Check sheet for the modelled part. Datum: model origin and axes. Units: mm. A direction names the side the tool comes from. Round coordinates to 2 decimals unless told otherwise and drop trailing zeros. Loops run counter-clockwise (first coordinate to the right, second up) from the corner with the lowest first, then second, coordinate; pieces in that order, holes last. Notation, with made-up numbers: (67, -28.5) - (81, -28.5) arc R19 cw to (81, -23.5) - close; hole circle Ø3 at (-17, 79). An arc over 180 degrees is marked (long way). Put each result on its own line as item: value.
```python
from build123d import *

# Parameters (mm, degrees)
BASE_FLANGE1_DEPTH      = 304.8
CUT_EXTRUDE1_DEPTH      = 408.166225608
CUT_EXTRUDE1_DEPTH_BACK = 408.166225608
SKETCH6_W               = 152.4
SKETCH6_H               = 12.7
EDGE_FLANGE1_DEPTH      = 521.87348
EDGE_FLANGE1_BEND_DEPTH = 521.87348
F_1_4_CLEARANCE_HOLE1_D = 6.7564
FILLET1_R               = 2.54
CUT_EXTRUDE2_DEPTH      = 412.498279143
CUT_EXTRUDE3_DEPTH      = 412.769633365
FILLET2_R               = 1.27


# Sheet-metal steps are written as plain solids
with BuildPart() as part:
    # Sketch1 → Base-Flange1 (new body)
    with BuildSketch(Plane(origin=(0, 0, 0), x_dir=(0, 0, -1), z_dir=(1, 0, 0))):
        with BuildLine():
            Line((-266.7, 44.45), (-266.7, 5.76326))
            ThreePointArc((-266.7, 5.76326), (-265.011980228, 1.688019772), (-260.93674, 0))
            Line((-260.93674, 0), (260.93674, 0))
            ThreePointArc((260.93674, 0), (265.011980228, 1.688019772), (266.7, 5.76326))
            Line((266.7, 5.76326), (266.7, 44.45))
            Line((266.7, 44.45), (264.11174, 44.45))
            Line((264.11174, 44.45), (264.11174, 5.76326))
            ThreePointArc((264.11174, 5.76326), (263.18180403, 3.51819597), (260.93674, 2.58826))
            Line((260.93674, 2.58826), (-260.93674, 2.58826))
            ThreePointArc((-260.93674, 2.58826), (-263.18180403, 3.51819597), (-264.11174, 5.76326))
            Line((-264.11174, 5.76326), (-264.11174, 44.45))
            Line((-264.11174, 44.45), (-266.7, 44.45))
        make_face()
    extrude(amount=BASE_FLANGE1_DEPTH)

    # Sketch6 → Cut-Extrude1 (cut, two sides: drawn at the far end of the back side and taken through both)
    with BuildSketch(Plane(origin=(0, 2.58826, 0), x_dir=(1, 0, 0), z_dir=(0, 1, 0)).offset(-CUT_EXTRUDE1_DEPTH_BACK)):
        with Locations((152.4, 260.35)):
            Rectangle(SKETCH6_W, SKETCH6_H)
        with Locations((152.4, -260.35)):
            Rectangle(SKETCH6_W, SKETCH6_H)
    extrude(amount=CUT_EXTRUDE1_DEPTH + CUT_EXTRUDE1_DEPTH_BACK, mode=Mode.SUBTRACT)

    # Edge-Flange1 section (across the edge) → Edge-Flange1 (add)
    with BuildSketch(Plane(origin=(-3.175, 2.58826, -260.93674), x_dir=(1, 0, 0), z_dir=(0, 0, 1))):
        with BuildLine():
            Line((-2.58826, 3.175), (-2.58826, 29.16174))
            Line((-2.58826, 29.16174), (0, 29.16174))
            Line((0, 29.16174), (0, 3.175))
            ThreePointArc((0, 3.175), (0.92993597, 0.92993597), (3.175, 0))
            Line((3.175, 0), (3.175, -2.58826))
            ThreePointArc((3.175, -2.58826), (-0.900240228, -0.900240228), (-2.58826, 3.175))
        make_face()
    extrude(amount=EDGE_FLANGE1_DEPTH)

    # Edge-Flange1 section 2 (across the edge) → Edge-Flange1 bend (add)
    with BuildSketch(Plane(origin=(307.975, 2.58826, 260.93674), x_dir=(-1, 0, 0), z_dir=(0, 0, -1))):
        with BuildLine():
            Line((-2.58826, 3.175), (-2.58826, 29.16174))
            Line((-2.58826, 29.16174), (0, 29.16174))
            Line((0, 29.16174), (0, 3.175))
            ThreePointArc((0, 3.175), (0.92993597, 0.92993597), (3.175, 0))
            Line((3.175, 0), (3.175, -2.58826))
            ThreePointArc((3.175, -2.58826), (-0.900240228, -0.900240228), (-2.58826, 3.175))
        make_face()
    extrude(amount=EDGE_FLANGE1_BEND_DEPTH)

    # 1/4 Clearance Hole1 (through all)
    with Locations(Plane.XY.offset(266.7)):
        with Locations((38.1, 31.75), (266.7, 31.75)):
            Hole(F_1_4_CLEARANCE_HOLE1_D / 2)

    # Fillet1
    fillet1_edges = [part.edges().sort_by_distance(p)[0] for p in [
        (0, 44.45, 265.40587),
        (-4.46913, 31.75, -260.93674),
        (-4.46913, 31.75, 260.93674),
        (0, 44.45, -265.40587),
        (309.26913, 31.75, 260.93674),
        (309.26913, 31.75, -260.93674),
        (304.8, 44.45, 265.40587),
        (76.2, 1.29413, -254),
        (228.6, 1.29413, -254),
        (228.6, 44.45, -265.40587),
        (76.2, 44.45, -265.40587),
        (304.8, 44.45, -265.40587),
        (228.6, 1.29413, 254),
        (76.2, 1.29413, 254),
        (76.2, 44.45, 265.40587),
        (228.6, 44.45, 265.40587),
    ]]
    fillet(fillet1_edges, radius=FILLET1_R)

    # Sketch15 → Cut-Extrude2 (cut, through all)
    with BuildSketch(Plane(origin=(0, 2.58826, 0), x_dir=(1, 0, 0), z_dir=(0, 1, 0))):
        with BuildLine():
            Line((149.86, 22.86), (149.86, 2.54))
            Line((149.86, 2.54), (129.54, 2.54))
            ThreePointArc((129.54, 2.54), (127, 0), (129.54, -2.54))
            Line((129.54, -2.54), (149.86, -2.54))
            Line((149.86, -2.54), (149.86, -22.86))
            ThreePointArc((149.86, -22.86), (152.4, -25.4), (154.94, -22.86))
            Line((154.94, -22.86), (154.94, -2.54))
            Line((154.94, -2.54), (175.26, -2.54))
            ThreePointArc((175.26, -2.54), (177.8, 0), (175.26, 2.54))
            Line((175.26, 2.54), (154.94, 2.54))
            Line((154.94, 2.54), (154.94, 22.86))
            ThreePointArc((154.94, 22.86), (152.4, 25.4), (149.86, 22.86))
        make_face()
    extrude(amount=-CUT_EXTRUDE2_DEPTH, mode=Mode.SUBTRACT)

    # Sketch16 → Cut-Extrude3 (cut, through all)
    with BuildSketch(Plane.XZ):
        with BuildLine():
            Line((149.86, -254), (149.86, -231.14))
            ThreePointArc((149.86, -231.14), (152.4, -228.6), (154.94, -231.14))
            Line((154.94, -231.14), (154.94, -254))
            Line((154.94, -254), (149.86, -254))
        make_face()
        with BuildLine():
            Line((154.94, 254), (149.86, 254))
            Line((149.86, 254), (149.86, 231.14))
            ThreePointArc((149.86, 231.14), (152.4, 228.6), (154.94, 231.14))
            Line((154.94, 231.14), (154.94, 254))
        make_face()
    extrude(amount=-CUT_EXTRUDE3_DEPTH, mode=Mode.SUBTRACT)

    # Fillet2
    fillet2_edges = [part.edges().sort_by_distance(p)[0] for p in [
        (149.86, 1.29413, -2.54),
        (154.94, 1.29413, -2.54),
        (154.94, 1.29413, 2.54),
        (149.86, 1.29413, 2.54),
        (154.94, 1.29413, 254),
        (149.86, 1.29413, 254),
        (154.94, 1.29413, -254),
        (149.86, 1.29413, -254),
    ]]
    fillet(fillet2_edges, radius=FILLET2_R)


solid = part.part
```
Item 1: Section check C-C on z = 221.5. Enter the section's corners in (x, y) (3 decimals), then the cut area to 3 significant figures.
Filled sheet:
outline: (-5.763, 5.763) arc R5.763 ccw to (0, 0) - (304.8, 0) arc R5.763 ccw to (310.563, 5.763) - (310.563, 31.75) - (307.975, 31.75) - (307.975, 5.763) arc R3.175 cw to (304.8, 2.588) - (0, 2.588) arc R3.175 cw to (-3.175, 5.763) - (-3.175, 31.75) - (-5.763, 31.75) - close
area: 960 mm²
Item 2: Thickness scan on line 1 (X direction, y = 27, z = -184.5) (3 decimals); line 2 (X direction, y = 31, z = 265); line 3 (Z direction, x = 68, y = 15). Record the ranges inside material, lowest first. Write a range as from..to.
Filled sheet:
line 1: -5.763..-3.175, 307.975..310.563
line 2: 0..34.81, 41.39..76.2, 228.6..263.41, 269.99..304.8
line 3: -266.7..-264.11, 264.11..266.7
Item 3: Tool access check on faces 5 (the flat face through (228.6, 18, 265)), 6 (the flat face through (-5.763, 19, -4)), 7 (the flat face through (307.975, 19, 4)), 8 (the flat face through (38, 25, 264.112)), 9 (the flat face through (76.2, 18, -265)). Record the directions out of +Z, -Z, +X, -X, +Y, -Y that give a thin tool (end or side, any length) a straight path to the whole face; none if there is none.
Filled sheet:
face 5: +Z, +Y, -Y
face 6: +Z, -Z, -X, +Y, -Y
face 7: +Z, -Z, +Y
face 8: +X, -X, +Y
face 9: -Z, +Y, -Y
Item 4: Section check A-A on y = 16.5. Enter the section's corners in (x, z) (3 decimals).
Filled sheet:
outline: (-5.763, -260.937) - (-3.175, -260.937) - (-3.175, 260.937) - (-5.763, 260.937) - close; (0, -266.7) - (76.2, -266.7) - (76.2, -264.112) - (0, -264.112) - close; (0, 264.112) - (76.2, 264.112) - (76.2, 266.7) - (0, 266.7) - close; (228.6, -266.7) - (304.8, -266.7) - (304.8, -264.112) - (228.6, -264.112) - close; (228.6, 264.112) - (304.8, 264.112) - (304.8, 266.7) - (228.6, 266.7) - close; (307.975, -260.937) - (310.563, -260.937) - (310.563, 260.937) - (307.975, 260.937) - close
Item 5: Section check D-D on x = 117.5. Enter the section's corners in (y, z).
Filled sheet:
outline: (0, -254) - (2.59, -254) - (2.59, 254) - (0, 254) - close
Item 6: Section check B-B on x = 239.5. Enter the section's corners in (y, z) (3 decimals), then the cut area to 3 significant figures.
Filled sheet:
outline: (0, -260.937) arc R5.763 ccw to (5.763, -266.7) - (44.45, -266.7) - (44.45, -264.112) - (5.763, -264.112) arc R3.175 cw to (2.588, -260.937) - (2.588, 260.937) arc R3.175 cw to (5.763, 264.112) - (44.45, 264.112) - (44.45, 266.7) - (5.763, 266.7) arc R5.763 ccw to (0, 260.937) - close
area: 1,590 mm²
Item 7: Release check for a two-part mould opening along Z. For faces 1 (the flat face through (184, 2.588, -4)), 2 (the flat face through (266, 25, -266.7)), 3 (the flat face through (-3.175, 19, -4)), 4 (the flat face through (266, 25, -264.112)) record: +Z half, -Z half, draft (parallel to the pull), parting line (faces both ways), or undercut.
Filled sheet:
face 1: undercut
face 2: -Z half
face 3: draft
face 4: undercut
Item 8: Go/stop test with flat-tipped pins: pin 1 (4 mm diameter, centred on x = 194.5, z = 104, fed in from +Y); pin 2 (3 mm diameter, centred on y = 2, z = 12, fed in from -X); pin 3 (3 mm diameter, centred on x = 143.5, y = 2, fed in from +Z). Record where each tip stops, or that it passes through.
Filled sheet:
pin 1: y = 2.59
pin 2: x = -5.3
pin 3: z = 254
